from build123d import *

# Parameters (mm, degrees)
ESQUISSE5_R             = 2.575
BOSS_EXTRU_2_DEPTH      = 7.8
ESQUISSE6_R             = 7.5
BOSS_EXTRU_3_DEPTH      = 20
BOSS_EXTRU_6_START      = -20
BOSS_EXTRU_6_DEPTH      = 20
ESQUISSE14_R            = 4.08
ENL_V_MAT_EXTRU_4_DEPTH = 48.235297536
ENL_V_MAT_EXTRU_5_DEPTH = 48.235297536
CONG_2_R                = 5
ESQUISSE17_R            = 2.05
ENL_V_MAT_EXTRU_6_DEPTH = 47.62863011
ENL_V_MAT_EXTRU_7_DEPTH = 3.25
ESQUISSE19_R            = 4.325
ENL_V_MAT_EXTRU_8_DEPTH = 5.5
ESQUISSE20_R            = 3.475
ENL_V_MAT_EXTRU_9_DEPTH = 4.97
CONG_3_R                = 2
CHANFREIN2_SIZE         = 2


with BuildPart() as part:
    # Esquisse5 → Boss.-Extru.2 (new body)
    with BuildSketch(Plane(origin=(0, 0, 0), x_dir=(1, 0, 0), z_dir=(0, 1, 0))):
        Polygon((-25, -14.43375673), (25, -14.43375673), (0, 28.867513459), align=None)
        with Locations(Location((0, 17, 0), (0, 0, 270))):
            Circle(ESQUISSE5_R, mode=Mode.SUBTRACT)
        with Locations(Location((-14.722431864, -8.5, 0), (0, 0, 270))):
            Circle(ESQUISSE5_R, mode=Mode.SUBTRACT)
        with Locations(Location((14.722431864, -8.5, 0), (0, 0, 270))):
            Circle(ESQUISSE5_R, mode=Mode.SUBTRACT)
    extrude(amount=BOSS_EXTRU_2_DEPTH)

    # Esquisse6 → Boss.-Extru.3 (add)
    with BuildSketch(Plane(origin=(0, 7.8, 0), x_dir=(1, 0, 0), z_dir=(0, 1, 0))):
        with Locations(Location((0, 0, 0), (0, 0, 270))):
            Circle(ESQUISSE6_R)
    extrude(amount=BOSS_EXTRU_3_DEPTH)

    # Esquisse13 → Boss.-Extru.6 (add)
    with BuildSketch(Plane(origin=(0, 27.8, 0), x_dir=(1, 0, 0), z_dir=(0, 1, 0)).offset(BOSS_EXTRU_6_START)):
        with BuildLine():
            Line((-7.5, 0), (-7.5, -14.43375673))
            Line((-7.5, -14.43375673), (7.5, -14.43375673))
            Line((7.5, -14.43375673), (7.5, 0))
            ThreePointArc((7.5, 0), (0, -7.5), (-7.5, 0))
        make_face()
    extrude(amount=BOSS_EXTRU_6_DEPTH)

    # Esquisse14 → Enlèv. mat.-Extru.4 (cut, through all)
    with BuildSketch(Plane(origin=(0, 27.8, 0), x_dir=(1, 0, 0), z_dir=(0, 1, 0))):
        with Locations(Location((0, 0, 0), (0, 0, 270))):
            Circle(ESQUISSE14_R)
    extrude(amount=-ENL_V_MAT_EXTRU_4_DEPTH, mode=Mode.SUBTRACT)

    # Esquisse15 → Enlèv. mat.-Extru.5 (cut, through all)
    with BuildSketch(Plane(origin=(0, 27.8, 0), x_dir=(1, 0, 0), z_dir=(0, 1, 0))):
        with BuildLine():
            Line((-1, -3.955553059), (-1, -14.43375673))
            Line((-1, -14.43375673), (1, -14.43375673))
            Line((1, -14.43375673), (1, -3.955553059))
            ThreePointArc((1, -3.955553059), (0, -4.08), (-1, -3.955553059))
        make_face()
    extrude(amount=-ENL_V_MAT_EXTRU_5_DEPTH, mode=Mode.SUBTRACT)

    # Congé2
    cong_2_edges = [part.edges().sort_by_distance(p)[0] for p in [
        (0, 3.9, -28.867513459),
        (25, 3.9, 14.43375673),
        (-25, 3.9, 14.43375673),
    ]]
    fillet(cong_2_edges, radius=CONG_2_R)

    # Esquisse17 → Enlèv. mat.-Extru.6 (cut, through all)
    with BuildSketch(Plane(origin=(7.5, 0, 0), x_dir=(0, 0, -1), z_dir=(1, 0, 0))):
        with Locations((-9.43375673, 20.3)):
            Circle(ESQUISSE17_R)
    extrude(amount=-ENL_V_MAT_EXTRU_6_DEPTH, mode=Mode.SUBTRACT)

    # Esquisse18 → Enlèv. mat.-Extru.7 (cut)
    with BuildSketch(Plane.ZY.offset(7.5)):
        Polygon((11.468916429, 23.825), (7.398597031, 23.825), (5.363437332, 20.3), (7.398597031, 16.775), (11.468916429, 16.775), (13.504076128, 20.3), align=None)
    extrude(amount=-ENL_V_MAT_EXTRU_7_DEPTH, mode=Mode.SUBTRACT)

    # Esquisse19 → Enlèv. mat.-Extru.8 (cut)
    with BuildSketch(Plane(origin=(0, 7.8, 0), x_dir=(1, 0, 0), z_dir=(0, 1, 0))):
        with Locations(Location((0, 17, 0), (0, 0, 270))):
            Circle(ESQUISSE19_R)
        with Locations(Location((14.722431864, -8.5, 0), (0, 0, 270))):
            Circle(ESQUISSE19_R)
        with Locations(Location((-14.722431864, -8.5, 0), (0, 0, 270))):
            Circle(ESQUISSE19_R)
    extrude(amount=-ENL_V_MAT_EXTRU_8_DEPTH, mode=Mode.SUBTRACT)

    # Esquisse20 → Enlèv. mat.-Extru.9 (cut)
    with BuildSketch(Plane(origin=(7.5, 0, 0), x_dir=(0, 0, -1), z_dir=(1, 0, 0))):
        with Locations((-9.43375673, 20.3)):
            Circle(ESQUISSE20_R)
    extrude(amount=-ENL_V_MAT_EXTRU_9_DEPTH, mode=Mode.SUBTRACT)

    # Congé3
    cong_3_edges = [part.edges().sort_by_distance(p)[0] for p in [
        (-4.25, 27.8, 14.43375673),
        (4.25, 27.8, 14.43375673),
    ]]
    fillet(cong_3_edges, radius=CONG_3_R)

    # Chanfrein2
    chanfrein2_edges = [part.edges().sort_by_distance(p)[0] for p in [
        (0, 7.8, -7.5),
        (7.5, 7.8, 7.216878365),
        (-7.5, 7.8, 7.216878365),
    ]]
    chamfer(chanfrein2_edges, length=CHANFREIN2_SIZE)


solid = part.part
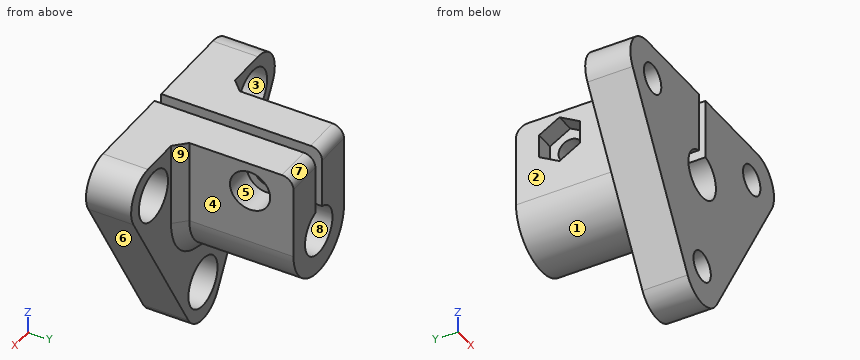
The listing builds one solid part. Answer for the finished solid, in the listing's coordinates (mm). Face numbers are marked on the shaded views. A direction names the side the tool comes from. Coordinates: 2 decimals unless noted, no trailing zeros. Order: outer loops, then holes, each group sorted by start corner. A loop starts at its lowest first (then second) coordinate and runs counter-clockwise, first axis right, second up. Notation, with made-up numbers: (45, 25) -> (99, 25) arc R12 cw to (99, 29) -> close; hole circle Ø3 at (47.25, 22). An arc over 180 degrees is marked (long way). Answer in a Markdown table with one row per item. Add a question column.
Item 1: Find section D-D (y = 3). Write down the section's boundary in (x, z) (3 decimals).
Item 2: Find section C-C (y = 9). Write down the section's boundary in (x, z), then the cut area to 3 significant figures.
Item 3: Find the intervals of material crossed by L1, parallel to Z at x = -2, y = 7.5; L2, parallel to X at y = 24.25, z = 6; L3, parallel to Z at x = -1.5, y = 4.5, in increasing order. Write a range as from..to.
Item 4: Which of the six approach directions +Z, -Z, +X, -X, +Y, -Y give full straight-line access (tool end or side, diameter ignored) to the marked faces 1, 2, 3, 4 and 5?
Item 5: Each of these flat-tipped pins is pushed along its axis until it touches: P1, Ø11.5, axis at y = 16.5, z = 4.5, coming from the -X side; P2, Ø5, axis at y = 4, z = 2.5, coming from the -X side; P3, Ø4.5, axis at x = 14.72, z = 8.5, coming from the +Y side; P4, Ø7, axis at y = 16.5, z = 5, coming from the +X side. Where does it stop, or does it pass through?
Item 6: Find section A-A (x = 0). Write down the section's boundary in (y, z) (3 decimals), then the cut area to 3 significant figures.
Item 7: Determine the mould class of the marked faces 6, 7, 8 and 9 for opening direction Z: +Z half, -Z half, draft (parallel to the pull), parting line (faces both ways), or undercut.
Item 8: Find section B-B (z = -17). Write down the section's boundary in (x, y) (3 decimals), then the cut area to 3 significant figures.
Result set:
| question | item | result |
|---|---|---|
| 1 | outline | (-20.67, 6.934) -> (-4.33, -21.368) arc R5 ccw to (4.33, -21.368) -> (20.67, 6.934) arc R5 ccw to (16.34, 14.434) -> (1, 14.434) -> (1, 3.956) arc R4.08 cw (long way) to (-1, 3.956) -> (-1, 14.434) -> (-16.34, 14.434) arc R5 ccw to start; hole circle Ø8.65 at (-14.722, 8.5); hole circle Ø8.65 at (0, -17); hole circle Ø8.65 at (14.722, 8.5) |
| 2 | outline | (-8.3, 0) arc R8.3 ccw to (8.3, 0) -> (8.3, 14.43) -> (1, 14.43) -> (1, 3.96) arc R4.08 cw (long way) to (-1, 3.96) -> (-1, 14.43) -> (-8.3, 14.43) -> close |
| 2 | area | 275 mm² |
| 3 | L1 | z = -23.45..-20.83, -13.17..-3.56, 3.56..14.43 |
| 3 | L2 | x = -7.5..-1, 1..7.5 |
| 3 | L3 | z = -23.64..-21.06, -12.94..-3.79, 3.79..14.43 |
| 4 | face 1 | -Z, +Y |
| 4 | face 2 | +Z, -Z, -X, +Y |
| 4 | face 3 | +Y |
| 4 | face 4 | +Z, -Z, +X, +Y |
| 4 | face 5 | +X |
| 5 | P1 | stops at x = -7.5 |
| 5 | P2 | stops at x = -19.55 |
| 5 | P3 | passes through |
| 5 | P4 | stops at x = 7.5 |
| 6 | outline | (0, -23.868) -> (7.8, -23.868) -> (7.8, -21.325) -> (2.3, -21.325) -> (2.3, -19.575) -> (0, -19.575) -> close; (0, -14.425) -> (2.3, -14.425) -> (2.3, -12.675) -> (7.8, -12.675) -> (7.8, -9.5) -> (9.8, -7.5) -> (27.8, -7.5) -> (27.8, -4.08) -> (0, -4.08) -> close |
| 6 | area | 165 mm² |
| 7 | face 6 | -Z half |
| 7 | face 7 | +Z half |
| 7 | face 8 | undercut |
| 7 | face 9 | draft |
| 8 | outline | (-6.852, 0) -> (-2.575, 0) -> (-2.575, 2.3) -> (-4.325, 2.3) -> (-4.325, 7.8) -> (-6.852, 7.8) -> close; (2.575, 0) -> (6.852, 0) -> (6.852, 7.8) -> (4.325, 7.8) -> (4.325, 2.3) -> (2.575, 2.3) -> close |
| 8 | area | 47.5 mm² |
